from build123d import *

# Parameters (mm, degrees)
F1_DEPTH = 3
F2_W     = 5
F2_H     = 50
F3_DEPTH = 3
F5_D     = 3
F8_D     = 3
F10_D    = 3
F12_D    = 3
F14_D    = 3


with BuildPart() as f1:
    # F0 (on Top) → F1 (new body)
    with BuildSketch(Plane.XY):
        Polygon((0, 10), (66, 0), (66, 143), (17, 163), (0, 163), align=None)
    extrude(amount=F1_DEPTH)

    # F2 (on face) → F3 (cut)
    with BuildSketch(Plane.XY.offset(3)):
        with Locations((58.5, 35)):
            Rectangle(F2_W, F2_H)
    extrude(amount=-F3_DEPTH, mode=Mode.SUBTRACT)

    # F5 (through all)
    with Locations(Plane.XY.offset(3)):
        with Locations((36, 19), (36, 51)):
            Hole(F5_D / 2)

    # F6: F1 across plane


with BuildPart() as f1_1:
    add(f1.part)
    add(f1.part.mirror(Plane.YZ))

    # F8 (through all)
    with Locations(Plane.XY.offset(3)):
        with Locations((0, 50)):
            Hole(F8_D / 2)

    # F10 (through all)
    with Locations(Plane.XY.offset(3)):
        with Locations((-37.773754, 87.5), (37.5, 87.5)):
            Hole(F10_D / 2)

    # F12 (through all)
    with Locations(Plane.XY.offset(3)):
        with Locations((37.5, 115)):
            Hole(F12_D / 2)

    # F14 (through all)
    with Locations(Plane.XY.offset(3)):
        with Locations((-10.5, 151.18438), (10.5, 151.18438)):
            Hole(F14_D / 2)


solid = f1_1.part
Geometry: final body of the model. Coordinates: model frame, mm. A direction names the side the tool comes from. Coordinates: 2 decimals unless noted, no trailing zeros. Order: outer loops, then holes, each group sorted by start corner. A loop starts at its lowest first (then second) coordinate and runs counter-clockwise, first axis right, second up. Notation, with made-up numbers: M 82.25,12 L 135.25,12 A23 cw 135.25,51 Z; hole C 31,77 d10. An arc over 180 degrees is marked long. One line per question, with ' | ' between items. Start each with the question number.
Item 1: Draft query along X for faces 3 (the flat face through (1, 83, 0)), 4 (the flat face through (33, 5, 1)), 5 (the flat face through (-41.84, 152.86, 1.48)). Return one class per face: released by +X, released by -X, zero draft, split by the parting line, or undercut.
Item 2: Pin query (flat end, axial travel): pin 1 Ø1.5 at (x, z) = (59.5, 1) entering from -Y; pin 2 Ø1.8 at (x, y) = (10.5, 151.18) entering from -Z; pin 3 Ø1.5 at (x, z) = (57.5, 1.5) entering from +Y. Return the tip coordinate at first contact, or that it passes through.
Item 3: Ray query, probe 1 along X at (y, z) = (55.5, 1.15); probe 2 along Y at (x, z) = (-36, 2.45); probe 3 along Y at (x, z) = (0, 1.75). Return the intervals inside material, ascending. Write a range as [from, to].
Item 4: Cut plane A-A, the plane y = 32. Return the cut outline in (x, z).
Item 5: Set-up query: faces 1 (the flat face through (-33, 5, 1)), 2 (the flat face through (1, 83, 3)). Return all of +Z, -Z, +X, -X, +Y, -Y with unobstructed straight access to the full face (end or side cutting, diameter ignored); none if empty.
Item 6: Cut plane C-C, the plane x = 28. Return the cut outline in (y, z).
Item 7: Cut plane B-B, the plane z = 1.05. Count the separate pieces of the cut face and the enclosed holes in it, then the cut area to 3 significant figures.
A:
1) face 3: zero draft | face 4: undercut | face 5: released by -X
2) pin 1: stops at y = 0.87 | pin 2: passes through | pin 3: stops at y = 146.78
3) probe 1: x = [-66, -61], [-56, 56], [61, 66] | probe 2: y = [4.55, 17.5], [20.5, 49.5], [52.5, 155.24] | probe 3: y = [10, 48.5], [51.5, 163]
4) outline: M -66,0 L -61,0 L -61,3 L -66,3 Z; M -56,0 L 56,0 L 56,3 L -56,3 Z; M 61,0 L 66,0 L 66,3 L 61,3 Z
5) face 1: +Z, -Z, -Y | face 2: +Z, +X, -X, +Y, -Y
6) outline: M 5.76,0 L 158.51,0 L 158.51,3 L 5.76,3 Z
7) separate pieces: 1 | enclosed holes: 12 | area: 19,300 mm2
